Check sheet for the drawn part. Datum: minimum x, y, z corner. Units: mm. A direction names the side the tool comes from. Round coordinates to 2 decimals unless told otherwise and drop trailing zeros. Order: outer loops, then holes, each group sorted by start corner. A loop starts at its lowest first (then second) coordinate and runs counter-clockwise, first axis right, second up. Notation, with made-up numbers: M 0.5,35 L 59.5,35 A24 cw 59.5,54 Z; hole C 72,5 d11. An arc over 180 degrees is marked long. Use one line per item in the form item = value. Start each with the question number.
Item 1: Thickness scan on probe 1 along Z at (x, y) = (7.5, 3.25); probe 2 along X at (y, z) = (1.75, 70.5); probe 3 along Y at (x, z) = (37, 34.5). Record the ranges inside material, lowest first. Write a range as [from, to].
Item 2: Cross-section at B-B on x = 30.5. Enter the section's corners in (y, z).
Item 3: Cross-section at A-A on z = 42. Enter the section's corners in (x, y), then the cut area to 3 significant figures.
Item 4: Go/stop test with flat-tipped pins: pin 1 Ø2 at (x, y) = (58, 5.5) entering from +Z; pin 2 Ø10 at (y, z) = (4, 34) entering from +X; pin 3 Ø8 at (x, y) = (75, 14.5) entering from +Z (3 decimals). Record where each tip stops, or that it passes through.
Item 5: Cross-section at C-C on y = 5.75. Enter the section's corners in (x, z), then the cut area to 3 significant figures.
Item 6: Cross-section at D-D on z = 20. Enter the section's corners in (x, y).
Item 7: Tool access check on the marked faces 1, 2, 3 and 4. Record the directions out of +Z, -Z, +X, -X, +Y, -Y that give a thin tool (end or side, any length) a straight path to the whole face; none if there is none.
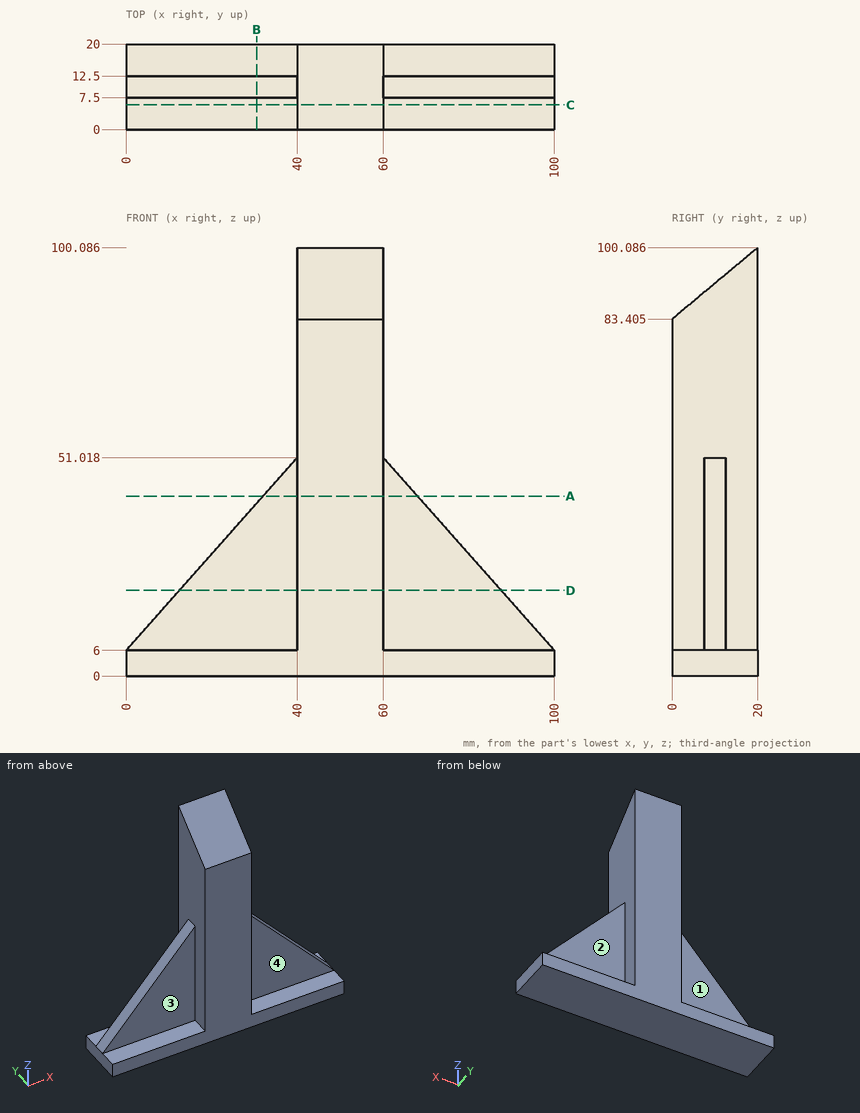
Output values:
q1.probe_1 = [0, 6]
q1.probe_2 = [40, 60]
q1.probe_3 = [7.5, 12.5]
q2.outline = M 0,0 L 20,0 L 20,6 L 12.5,6 L 12.5,40.33 L 7.5,40.33 L 7.5,6 L 0,6 Z
q3.outline = M 31.99,7.5 L 40,7.5 L 40,0 L 60,0 L 60,7.5 L 68.01,7.5 L 68.01,12.5 L 60,12.5 L 60,20 L 40,20 L 40,12.5 L 31.99,12.5 Z
q3.area = 480 mm2
q4.pin_1 = 88.83
q4.pin_2 = 78.29
q4.pin_3 = 38.035
q5.outline = M 0,0 L 100,0 L 100,6 L 60,6 L 60,88.2 L 40,88.2 L 40,6 L 0,6 Z
q5.area = 2,240 mm2
q6.outline = M 12.44,7.5 L 40,7.5 L 40,0 L 60,0 L 60,7.5 L 87.56,7.5 L 87.56,12.5 L 60,12.5 L 60,20 L 40,20 L 40,12.5 L 12.44,12.5 Z
q7.face_1 = +Z, -X, +Y
q7.face_2 = +Z, +X, +Y
q7.face_3 = +Z, -X, -Y
q7.face_4 = +Z, +X, -Y
